Geometry check sheet. Reference: the model listing, model coordinates, mm. A direction names the side the tool comes from. Give positions to 0.01 mm unless a question says otherwise; leave off trailing zeros. Loops run counter-clockwise (first coordinate to the right, second up) from the corner with the lowest first, then second, coordinate; pieces in that order, holes last. Notation, with made-up numbers: (51.25, 10) -> (81.25, 10) arc R20 cw to (81.25, 34) -> close; hole circle Ø7 at (87.5, -25). An arc over 180 degrees is marked (long way). Answer in a Markdown table with one row per item. Add a question column.
```python
from build123d import *

# Parameters (mm, degrees)
F0_R     = 10
F1_DEPTH = 60
F2_R     = 20
F2_R_2   = 10
F3_DEPTH = 3
F4_SIZE  = 2
F6_D     = 6.5
F7_SIZE  = 0.5


with BuildPart() as f1:
    # F0 (on Front) → F1 (new body)
    with BuildSketch(Plane.XZ):
        Circle(F0_R)
    extrude(amount=F1_DEPTH)

    # F2 (on face) → F3 (join)
    with BuildSketch(Plane(origin=(0, 0, 0), x_dir=(-1, 0, 0), z_dir=(0, 1, 0))):
        Circle(F2_R)
        Circle(F2_R_2, mode=Mode.SUBTRACT)
        Circle(F2_R_2)
    extrude(amount=F3_DEPTH)

    # F4
    f4_edges = [f1.edges().sort_by_distance(p)[0] for p in [
        (-10, -60, 0),
    ]]
    chamfer(f4_edges, length=F4_SIZE)

    # F6 (through all)
    with Locations(Plane(origin=(0, 3, 0), x_dir=(-1, 0, 0), z_dir=(0, 1, 0))):
        with Locations((0, 15)):
            Hole(F6_D / 2)

    # F7
    f7_edges = [f1.edges().sort_by_distance(p)[0] for p in [
        (20, 3, 0),
    ]]
    chamfer(f7_edges, length=F7_SIZE)


solid = f1.part
```
1. Sectioned sample at A-A (x = 0). Enter the section's corners in (y, z).
2. Access from +Z, -Z, +X, -X, +Y, -Y to the whole of each face (thin tool, end or side, straight path). Record for faces 1 (the face through (0, -60, 0)), 2 (the face through (-2.17, -28.59, -9.76)).
3. Release check for a two-part mould opening along X. For faces 3 (the face through (-0.423, 1.479, 18.222)), 4 (the face through (4.336, 1.232, -19.524)), 5 (the face through (9, 0, 5)) record: released by +X, released by -X, zero draft, split by the parting line, or undercut.
4. Gauge pin test, flat ends, axial feed: pin 1 Ø4 at (y, z) = (-53.5, 7.5) entering from +X; pin 2 Ø8 at (x, y) = (-11, -22.5) entering from -Z; pin 3 Ø12 at (x, y) = (-8, -29) entering from +Z. Record the tip position at first contact, or that the pin passes through.
5. Sectioned sample at B-B (z = 0). Enter the section's corners in (x, y), plus the area to 3 significant figures.
6. Material ranges on L1, parallel to Z at x = 0, y = 2.15; L2, parallel to Y at x = -16, z = 11; L3, parallel to Z at x = -0.5, y = -26.5, recorded low to high. Write a range as from..to.
7. Sectioned sample at C-C (y = -3). Enter the section's corners in (x, z).
Response:
| question | item | result |
|---|---|---|
| 1 | outline | (-60, -8) -> (-58, -10) -> (0, -10) -> (0, -20) -> (2.5, -20) -> (3, -19.5) -> (3, 11.75) -> (0, 11.75) -> (0, 10) -> (-58, 10) -> (-60, 8) -> close; (0, 18.25) -> (3, 18.25) -> (3, 19.5) -> (2.5, 20) -> (0, 20) -> close |
| 2 | face 1 | +Z, -Z, +X, -X, -Y |
| 2 | face 2 | -Y |
| 3 | face 3 | undercut |
| 3 | face 4 | split by the parting line |
| 3 | face 5 | zero draft |
| 4 | pin 1 | stops at x = 8.35 |
| 4 | pin 2 | stops at z = -7.14 |
| 4 | pin 3 | stops at z = 9.8 |
| 5 | outline | (-20, 0) -> (-10, 0) -> (-10, -58) -> (-8, -60) -> (8, -60) -> (10, -58) -> (10, 0) -> (20, 0) -> (20, 2.5) -> (19.5, 3) -> (-19.5, 3) -> (-20, 2.5) -> close |
| 5 | area | 1,320 mm2 |
| 6 | L1 | z = -20..11.75, 18.25..20 |
| 6 | L2 | y = 0..3 |
| 6 | L3 | z = -9.99..9.99 |
| 7 | outline | circle Ø20 at (0, 0) |
